Build history of the part. All positions in model axes, mm. Face numbers are marked on the shaded views. A direction names the side the tool comes from. Coordinates: 2 decimals unless noted, no trailing zeros. Order: outer loops, then holes, each group sorted by start corner. A loop starts at its lowest first (then second) coordinate and runs counter-clockwise, first axis right, second up. Notation, with made-up numbers: (-29.5, 67) - (-3.5, 67) arc R11 ccw to (-3.5, 85) - close; hole circle Ø6 at (-6.75, 84.5). An arc over 180 degrees is marked (long way). Answer as CSV lines item,"result". Start each with the question number.
Autodesk Fusion 360 part; units mm, degrees
box "BoxPrimitive1" add length 70 width 74 height 20 placed x (0, -1, 0) y (1, 0, 0) z (0, 0, 1) at (-30, 30, 0)
sketch "Sketch2" plane through (0, 0, 20) normal (0, 0, 1) x (-1, 0, 0)
  line L0 (30, 40) -> (-44, 40)
  line L1 (-44, 40) -> (-44, -30)
  line L2 (-44, -30) -> (30, -30)
  line L3 (30, -30) -> (30, 40)
  circle A0 centre (12, -15) radius 7.5
  circle A1 centre (12, 25) radius 7.5
  point P0 (30, -15)
  point P1 (30, 25)
  point P2 (12, -30)
  point P3 (12, -15)
  point P4 (12, 25)
  dimension "d9" = 15
  dimension "d10" = 15
extrude "Extrude1" cut sketch "Sketch2" against normal blind 378 contours A0 | A1
sketch "Sketch3" plane through (0, 0, 0) normal (0, 0, -1) x (1, 0, 0)
  circle A0 centre (-12, -15) radius 7.5
  circle A1 centre (-12, 25) radius 7.5
  line L0 (44, 40) -> (-30, 40)
  line L1 (-30, 40) -> (-30, -30)
  line L2 (-30, -30) -> (44, -30)
  line L3 (44, -30) -> (44, 40)
  line L4 (-0.5, 25) -> (-0.5, 40)
  line L5 (-0.5, 40) -> (-23.5, 40)
  line L6 (-23.5, 40) -> (-23.5, 25)
  line L7 (-23.5, -15) -> (-23.5, -30)
  line L8 (-23.5, -30) -> (-0.5, -30)
  line L9 (-0.5, -30) -> (-0.5, -15)
  arc A2 (-0.5, -15) -> (-23.5, -15) centre (-12, -15) ccw
  arc A3 (-23.5, 25) -> (-0.5, 25) centre (-12, 25) ccw
  dimension "d13" = 23
  dimension "d14" = 23
  dimension "d15" = 23
  dimension "d16" = 23
extrude "Extrude2" cut sketch "Sketch3" against normal blind 12 contours L0 L4 L5 L6 A3 | L2 L7 L8 L9 A2
sketch "Sketch4" plane through (0, 0, 20) normal (0, 0, 1) x (-1, 0, 0)
  circle A0 centre (12, -15) radius 7.5
  circle A1 centre (12, 25) radius 7.5
  line L0 (30, 40) -> (-44, 40)
  line L1 (-44, -30) -> (30, -30)
  line L2 (30, -30) -> (30, 40)
  circle A2 centre (-44, 5) radius 35
  point P0 (-44, 5)
extrude "Extrude3" add sketch "Sketch4" along normal blind 15 and the other way blind 20 contours A2
sketch "Sketch5" plane through (0, 0, 35) normal (0, 0, 1) x (-1, 0, 0)
  circle A0 centre (-44, 5) radius 35
sketch "Sketch6" plane through (0, 0, 35) normal (0, 0, 1) x (-1, 0, 0)
  circle A0 centre (-44, 5) radius 35
  dimension "d23" = 70
sphere "SpherePrimitive1" add diameter 70 placed x (-1, 0, 0) y (0, -1, 0) z (0, 0, 1) at (44, -5, 35)
sketch "Sketch8" plane through (0, 30, 0) normal (0, 1, 0) x (-1, 0, 0)
  line L0 (0.5, 0) -> (0.5, 12)
  line L1 (0.5, 12) -> (23.5, 12)
  line L2 (23.5, 12) -> (23.5, 0)
  line L3 (23.5, 0) -> (30, 0)
  line L4 (30, 0) -> (30, 20)
  line L5 (30, 20) -> (-44, 20)
  line L6 (-44, 20) -> (-44, 0)
  line L7 (-44, 0) -> (0.5, 0)
  line L8 (-34, 50) -> (-54, 50)
  line L9 (-54, 50) -> (-54, 30)
  line L10 (-54, 30) -> (-34, 30)
  line L11 (-34, 30) -> (-34, 50)
  line L12 (-34, 50) -> (-54, 30) construction
  line L13 (-54, 50) -> (-34, 30) construction
  point P0 (-44, 40)
  point P1 (-44, 40)
  dimension "d26" = 20
  dimension "d27" = 20
extrude "Extrude4" cut sketch "Sketch8" against normal blind 15 contours L8 L9 L10 L11
sketch "Sketch9" plane through (0, 0, 0) normal (0, 0, -1) x (1, 0, 0)
  line L0 (44, 40) -> (-0.5, 40)
  line L1 (-0.5, 40) -> (-0.5, 25)
  arc A0 (-23.5, 25) -> (-0.5, 25) centre (-12, 25) ccw
  line L2 (-23.5, 25) -> (-23.5, 40)
  line L3 (-23.5, 40) -> (-30, 40)
  line L4 (-30, 40) -> (-30, -30)
  line L5 (-30, -30) -> (-23.5, -30)
  line L6 (-23.5, -30) -> (-23.5, -15)
  arc A1 (-0.5, -15) -> (-23.5, -15) centre (-12, -15) ccw
  line L7 (-0.5, -15) -> (-0.5, -30)
  line L8 (-0.5, -30) -> (44, -30)
  arc A2 (44, -30) -> (44, 40) centre (44, 5) ccw
  circle A3 centre (44, 5) radius 28
extrude "Extrude5" cut sketch "Sketch9" against normal blind 35 contours A3
sketch "Sketch10" plane through (0, 0, 35) normal (0, 0, -1) x (1, 0, 0)
  line L0 (34, -21.1534) -> (34, -15)
  line L1 (34, -15) -> (54, -15)
  line L2 (54, -15) -> (54, -21.1534)
  arc A0 (54, -21.1534) -> (34, -21.1534) centre (44, 5) ccw
  circle A1 centre (44, 5) radius 28
sphere "SpherePrimitive2" cut diameter 56 placed x (1, 0, 0) y (0, -1, 0) z (0, 0, -1) at (44, -5, 35)
sketch "Sketch12" plane through (0, 0, 20) normal (0, 0, 1) x (-1, 0, 0)
  arc A0 (-44, -30) -> (-44, 40) centre (-44, 5) ccw
  line L0 (-44, -30) -> (30, -30)
  line L1 (30, -30) -> (30, 40)
  line L2 (30, 40) -> (-44, 40)
  circle A1 centre (12, -15) radius 7.5
  circle A2 centre (12, 25) radius 7.5
  line L3 (12, 5) -> (12, -2)
  line L4 (12, -2) -> (12, 5)
  line L5 (12, 5) -> (12, 12)
  line L6 (12, -2) -> (-11.2915, -2)
  line L7 (-11.2915, -2) -> (-11.2915, 12)
  line L8 (-11.2915, 12) -> (12, 12)
  point P0 (30, 5)
extrude "Extrude6" add sketch "Sketch12" along normal blind 15 contours A0 L6 L7 L8 | A0 L3 L4 L5 L6 L8
sketch "Sketch13" plane through (0, 2, 0) normal (0, 1, 0) x (-1, 0, 0)
  line L0 (-9.7071, 35) -> (-9.7071, 20)
  line L1 (-9.7071, 20) -> (12, 20)
  line L2 (12, 20) -> (12, 35)
  line L3 (12, 35) -> (-9.7071, 35)
  line L4 (12, 20) -> (-10, 35)
extrude "Extrude7" cut sketch "Sketch13" against normal blind 20 contours L0 L2 L3 L4
sketch "Sketch14" plane through (0, 0, 0) normal (0, 0, -1) x (1, 0, 0)
  circle A0 centre (44, 5) radius 28
  line L0 (44, 40) -> (-0.5, 40)
  line L1 (-0.5, 40) -> (-0.5, 25)
  arc A1 (-23.5, 25) -> (-0.5, 25) centre (-12, 25) ccw
  line L2 (-23.5, 25) -> (-23.5, 40)
  line L3 (-23.5, 40) -> (-30, 40)
  line L4 (-30, 40) -> (-30, -30)
  line L5 (-30, -30) -> (-23.5, -30)
  line L6 (-23.5, -30) -> (-23.5, -15)
  arc A2 (-0.5, -15) -> (-23.5, -15) centre (-12, -15) ccw
  line L7 (-0.5, -15) -> (-0.5, -30)
  line L8 (-0.5, -30) -> (44, -30)
  arc A3 (44, -30) -> (44, 40) centre (44, 5) ccw
  line L9 (-30, 5) -> (79, 5)
  line L10 (79, 5) -> (90, 5)
  line L11 (90, 5) -> (90, 19)
  line L12 (90, 19) -> (90, 5)
  line L13 (90, 5) -> (90, -9)
  line L14 (90, -9) -> (73.8174, -9)
  line L15 (73.8174, -9) -> (73.8174, 19)
  line L16 (73.8174, 19) -> (90, 19)
  line L17 (90, 19) -> (90, -9)
extrude "Extrude8" add sketch "Sketch14" against normal blind 35 contours A3 L9 L15 L16 | A3 L9 L14 L15 | A3 L10 L13 L14 L17 | A3 L10 L11 L12 L16 L17
sketch "Sketch15" plane through (90, 0, 0) normal (1, 0, 0) x (0, 1, 0)
  line L0 (-19, 0) -> (9, 0)
  line L1 (9, 0) -> (9, 35)
  line L2 (9, 35) -> (-19, 35)
  line L3 (-19, 35) -> (-19, 0)
  line L4 (-5, 0) -> (-14, 0)
  line L5 (-5, 0) -> (4, 0)
  line L6 (-14, 0) -> (4, 0)
  line L7 (4, 0) -> (4, 30)
  line L8 (4, 30) -> (-14, 30)
  line L9 (-14, 30) -> (-14, 0)
  point P0 (-5, 0)
  dimension "d48" = 30
extrude "Extrude9" cut sketch "Sketch15" against normal blind 21 contours L0 L4 L5 L6 L7 L8 L9
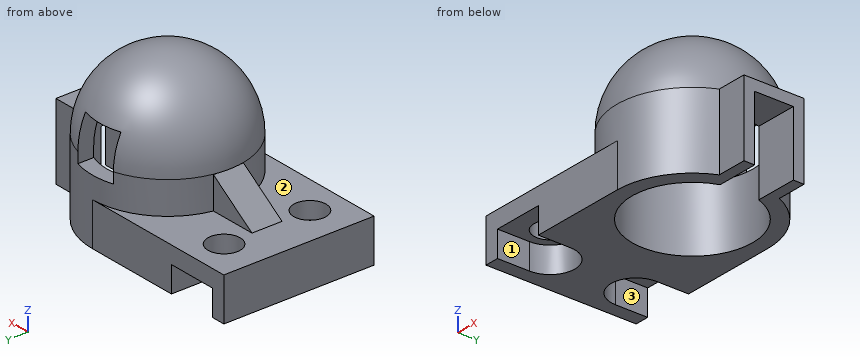
(1) Band-saw the part on D-D on z = 27. List the corners of the cut face in (x, y), plus the area to 3 significant figures.
(2) Which spindle directions (+Z, -Z, +X, -X, +Y, -Y) get a long thin tool onto all of the face, cutting with end or side? Do the marked faces 1, 2 and 3. Say none if no direction does.
(3) Probe L1, parallel to Y at x = -12, z = 18; L2, parallel to Y at x = 44, z = 20.5; L3, parallel to X at y = 15, z = 17.75. List the from-to ranges inside material, lowest first. Write a range as [from, to].
(4) Band-saw the part on B-B on y = -5. List the corners of the cut face in (x, z).
(5) Band-saw the part on C-C on x = 31. List the corners of the cut face in (y, z), plus the area to 3 significant figures.
(6) Drop flat-ended pins along their axis: pin 1 Ø7.5 at (x, z) = (2, 27.5) entering from +Y; pin 2 Ø12 at (x, z) = (3, 27) entering from -Y; pin 3 Ø8 at (y, z) = (14, 44) entering from -X; pin 4 Ø10 at (x, y) = (64.5, -29) entering from -Z. Give the stop position or say it passes through.
(7) Band-saw the part on A-A on y = 18.5. List the corners of the cut face in (x, z), plus the area to 3 significant figures.
Filled in:
1,outline,"(-1.73, -12) - (9.71, -12) arc R35 ccw to (76.08, -19) - (90, -19) - (90, -14) - (70.51, -14) arc R28 cw (long way) to (70.51, 4) - (90, 4) - (90, 9) - (76.08, 9) arc R35 ccw to (9.71, 2) - (-1.73, 2) - close"
1,area,"1,540 mm^2"
2,face 1,"-Z, -Y"
2,face 2,"+Z, -X"
2,face 3,"-Z, +Y"
3,L1,"y = [-40, -32.5], [-17.5, 7.5], [22.5, 30]"
3,L2,"y = [-40, -33], [23, 30]"
3,L3,"x = [-30, -19.5], [-4.5, 24.4], [63.6, 72.72]"
4,outline,"(-30, 0) - (16, 0) - (16, 35) arc R28 cw to (72, 35) - (72, 30) - (90, 30) - (90, 35) - (79, 35) arc R35 ccw to (9, 35) - (9.71, 35) - (9.71, 34.8) - (-12, 20) - (-30, 20) - close"
5,outline,"(-40, 0) - (-29.8, 0) - (-29.8, 35) arc R24.8 cw to (19.8, 35) - (19.8, 0) - (30, 0) - (30, 20) - (27.5, 20) - (27.5, 35) arc R32.5 ccw to (-37.5, 35) - (-37.5, 20) - (-40, 20) - close"
5,area,"1,330 mm^2"
6,pin 1,"stops at y = 2"
6,pin 2,"stops at y = -12"
6,pin 3,"stops at x = 13.42"
6,pin 4,"stops at z = 0"
7,outline,"(-30, 0) - (-23.5, 0) - (-23.5, 12) - (-18.63, 12) - (-18.63, 20) - (-30, 20) - close; (-5.37, 12) - (-0.5, 12) - (-0.5, 0) - (28.78, 0) - (28.78, 35) arc R15.22 cw to (34, 46.48) - (34, 50) - (41.4, 50) arc R15.22 cw to (46.6, 50) - (54, 50) - (54, 46.48) arc R15.22 cw to (59.22, 35) - (59.22, 0) - (69.94, 0) - (69.94, 35) arc R25.94 ccw to (18.06, 35) - (18.06, 20) - (-5.37, 20) - close"
7,area,"2,000 mm^2"
